The listing builds one solid part. Answer for the finished solid, in the listing's coordinates (mm). Give positions to 0.01 mm unless a question says otherwise; leave off trailing zeros. Write each loop counter-clockwise with the first axis right and the second up, starting at its lowest first coordinate (ties: lowest second). Pieces come first, ordered by that corner, then holes. Notation, with made-up numbers: (51.5, 34.5) - (106.5, 34.5) arc R20 ccw to (106.5, 57.5) - close; hole circle Ø9 at (59.25, 5.5). An arc over 180 degrees is marked (long way). One line per question, with ' | ' between items. Start each with the question number.
1. Find the intervals of material crossed by L1, parallel to Z at x = 0, y = -3; L2, parallel to X at y = -5.05, z = -1.5; L3, parallel to X at y = -3.9, z = 0.5, in increasing order. Write a range as from..to.
2. A cutting plane is placed at D-D (y = -0.6). Determine the outline of the cut face in (x, z), then the cut area to 3 significant figures.
3. Given P1, Ø1, axis at x = 7.5, z = -6.5, coming from the +Y side; P2, Ø1.5, axis at y = -1, z = -1.5, coming from the -X side; P3, Ø3, axis at x = 8, z = 0.5, coming from the +Y side (3 decimals); P4, Ø1.5, axis at y = -3, z = 2.5, coming from the -X side, each flat-ended and moving along its own axis, determine where each tip first touches the part or whether it passes through.
4. A cutting plane is placed at C-C (y = -3.2). Determine the outline of the cut face in (x, z).
```python
from build123d import *

# Parameters (mm, degrees)
F0_R     = 12.15
F0_R_2   = 10.15
F1_DEPTH = 6
F2_R     = 1
F3_R     = 0.99999


# Not quite as in the source:
# - a fillet or chamfer is up to 0.001 mm smaller than in the source, because OpenCascade refuses the exact size


with BuildPart() as f1:
    # F0 (on Front) → F1 (new body)
    with BuildSketch(Plane.XZ):
        Circle(F0_R)
        Circle(F0_R_2, mode=Mode.SUBTRACT)
    extrude(amount=F1_DEPTH)

    # F2
    f2_edges = [f1.edges().sort_by_distance(p)[0] for p in [
        (-10.15, -6, 0),
        (-10.15, 0, 0),
    ]]
    fillet(f2_edges, radius=F2_R)

    # F3 (radius 1 in the source; OpenCascade refuses exactly that, so slightly less here)
    f3_edges = [f1.edges().sort_by_distance(p)[0] for p in [
        (-12.15, 0, 0),
        (-12.15, -6, 0),
    ]]
    fillet(f3_edges, radius=F3_R)


solid = f1.part
```
Determined:
1) L1: -12.15..-10.15, 10.15..12.15 | L2: -12.06..-10.04, 10.04..12.06 | L3: -12.14..-10.14, 10.14..12.14
2) outline: circle Ø24.13 at (0, 0); hole circle Ø20.47 at (0, 0) | area: 128 mm2
3) P1: y = -0.31 | P2: x = -12.13 | P3: through | P4: x = -12.02
4) outline: circle Ø24.3 at (0, 0); hole circle Ø20.3 at (0, 0)
